Source: CAD feature listing. Evaluate the final solid. Frame: model axes, mm. A direction names the side the tool comes from. Give positions to 0.01 mm unless a question says otherwise; leave off trailing zeros. Write each loop counter-clockwise with the first axis right and the second up, starting at its lowest first coordinate (ties: lowest second). Pieces come first, ordered by that corner, then holes. Notation, with made-up numbers: M 47.25,20 L 69.25,20 A18 cw 69.25,49 Z; hole C 50,7.25 d5. An arc over 180 degrees is marked long. Answer as a JSON object with one key per item and string values. Group by question number.
```python
from build123d import *

# Parameters (mm, degrees)
F0_R          = 5.5
F0_R_2        = 5
F2_DEPTH      = 4
F3_W          = 37.252
F3_H          = 4.7996
F4_DEPTH      = 7.025
F4_DEPTH_BACK = 7.025
F5_T4_DEPTH   = 25.1150634776
F5_T10_DEPTH  = 25.1150634776
F5_T16_DEPTH  = 25.8484060864
F5_T22_DEPTH  = 25.8484060864


# Not quite as in the source:
# - a fillet or chamfer that OpenCascade refuses, or shapes differently, is made with other operations: its cross-section is extruded or revolved along the edge and cut away or added


with BuildPart() as f2:
    # F0 (on Top) → F2 (new body, symmetric)
    with BuildSketch(Plane.XY):
        with BuildLine():
            ThreePointArc((-25.4642125984, 6.5236839855), (-20.8095940807, 4.6358116329), (-18.876, 0))
            ThreePointArc((-18.876, 0), (-20.8095940807, -4.6358116329), (-25.4642125984, -6.5236839855))
            Line((-25.4642125984, -6.5236839855), (25.3308661417, -7.0236597661))
            ThreePointArc((25.3308661417, -7.0236597661), (18.376, 0), (25.3308661417, 7.0236597661))
            Line((25.3308661417, 7.0236597661), (-25.4642125984, 6.5236839855))
        make_face()
        with BuildLine():
            ThreePointArc((32.424, 0), (30.3422150793, 4.9911006913), (25.3308661417, 7.0236597661))
            ThreePointArc((25.3308661417, 7.0236597661), (18.376, 0), (25.3308661417, -7.0236597661))
            ThreePointArc((25.3308661417, -7.0236597661), (30.3422150793, -4.9911006913), (32.424, 0))
        make_face()
        with Locations((25.4, 0)):
            Circle(F0_R, mode=Mode.SUBTRACT)
        with BuildLine():
            ThreePointArc((-25.4642125984, -6.5236839855), (-20.8095940807, -4.6358116329), (-18.876, 0))
            ThreePointArc((-18.876, 0), (-20.8095940807, 4.6358116329), (-25.4642125984, 6.5236839855))
            ThreePointArc((-25.4642125984, 6.5236839855), (-31.924, 0), (-25.4642125984, -6.5236839855))
        make_face()
        with Locations((-25.4, 0)):
            Circle(F0_R_2, mode=Mode.SUBTRACT)
    extrude(amount=F2_DEPTH, both=True)

    # F3 (on Front) → F4 (cut, two sides)
    with BuildSketch(Plane.XZ) as f4_sk:
        with Locations((-0.25, 0)):
            Rectangle(F3_W, F3_H)
    extrude(amount=-F4_DEPTH, mode=Mode.SUBTRACT)
    extrude(f4_sk.sketch, amount=F4_DEPTH_BACK, mode=Mode.SUBTRACT)

    # F5: fillet of radius 2.3876 on 4 edges, made by hand


with BuildPart() as f5_tool2:
    # F5_s3 → F5_t4 (new body)
    with BuildSketch(Plane.XZ.offset(-12.5575317388)):
        with BuildLine():
            ThreePointArc((-18.876, 0.0122), (-18.1766881508, 1.7004881508), (-16.4884, 2.3998))
            Line((-16.4884, 2.3998), (-18.876, 2.3998))
            Line((-18.876, 2.3998), (-18.876, 0.0122))
        make_face()
    extrude(amount=F5_T4_DEPTH)

    split(bisect_by=Plane(origin=(-0.0666732283, 6.7736718758, 0), x_dir=(0, 0, 1), z_dir=(0.0098425197, -0.9999515612, 0)), keep=Keep.TOP)

    split(bisect_by=Plane(origin=(-0.0666732283, -6.7736718758, 0), x_dir=(0, 0, 1), z_dir=(0.0098425197, 0.9999515612, 0)), keep=Keep.TOP)


with BuildPart() as f2_1:
    add(f2.part)

    # F5_t1: union F5_tool2
    add(f5_tool2.part)


with BuildPart() as f5_tool8:
    # F5_s9 → F5_t10 (new body)
    with BuildSketch(Plane.XZ.offset(12.5575317388)):
        with BuildLine():
            ThreePointArc((-16.4884, -2.3998), (-18.1766881508, -1.7004881508), (-18.876, -0.0122))
            Line((-18.876, -0.0122), (-18.876, -2.3998))
            Line((-18.876, -2.3998), (-16.4884, -2.3998))
        make_face()
    extrude(amount=-F5_T10_DEPTH)

    split(bisect_by=Plane(origin=(-0.0666732283, 6.7736718758, 0), x_dir=(0, 0, 1), z_dir=(0.0098425197, -0.9999515612, 0)), keep=Keep.TOP)

    split(bisect_by=Plane(origin=(-0.0666732283, -6.7736718758, 0), x_dir=(0, 0, 1), z_dir=(0.0098425197, 0.9999515612, 0)), keep=Keep.TOP)


with BuildPart() as f2_2:
    add(f2_1.part)

    # F5_t7: union F5_tool8
    add(f5_tool8.part)


with BuildPart() as f5_tool14:
    # F5_s15 → F5_t16 (new body)
    with BuildSketch(Plane.XZ.offset(12.9242030432)):
        with BuildLine():
            ThreePointArc((18.376, -0.0122), (17.6766881508, -1.7004881508), (15.9884, -2.3998))
            Line((15.9884, -2.3998), (18.376, -2.3998))
            Line((18.376, -2.3998), (18.376, -0.0122))
        make_face()
    extrude(amount=-F5_T16_DEPTH)

    split(bisect_by=Plane(origin=(-0.0666732283, 6.7736718758, 0), x_dir=(0, 0, 1), z_dir=(0.0098425197, -0.9999515612, 0)), keep=Keep.TOP)

    split(bisect_by=Plane(origin=(-0.0666732283, -6.7736718758, 0), x_dir=(0, 0, 1), z_dir=(0.0098425197, 0.9999515612, 0)), keep=Keep.TOP)


with BuildPart() as f2_3:
    add(f2_2.part)

    # F5_t13: union F5_tool14
    add(f5_tool14.part)


with BuildPart() as f5_tool20:
    # F5_s21 → F5_t22 (new body)
    with BuildSketch(Plane.XZ.offset(-12.9242030432)):
        with BuildLine():
            ThreePointArc((18.376, 0.0122), (17.6766881508, 1.7004881508), (15.9884, 2.3998))
            Line((15.9884, 2.3998), (18.376, 2.3998))
            Line((18.376, 2.3998), (18.376, 0.0122))
        make_face()
    extrude(amount=F5_T22_DEPTH)

    split(bisect_by=Plane(origin=(-0.0666732283, 6.7736718758, 0), x_dir=(0, 0, 1), z_dir=(0.0098425197, -0.9999515612, 0)), keep=Keep.TOP)

    split(bisect_by=Plane(origin=(-0.0666732283, -6.7736718758, 0), x_dir=(0, 0, 1), z_dir=(0.0098425197, 0.9999515612, 0)), keep=Keep.TOP)


with BuildPart() as f2_4:
    add(f2_3.part)

    # F5_t19: union F5_tool20
    add(f5_tool20.part)


solid = f2_4.part
```
(1) Pull-direction query (X, two-part tool) for faces 3 (the cylindrical face through (-31.922, 0.143, 0.056)), 4 (the flat face through (0, 0, 4)), 5 (the cylindrical face through (-30.395, 0.22, -0.056)); classes: pulls with the +X half, pulls with the -X half, needs draft (parallel to the pull), parting line crosses it, or undercut.
(2) Section C-C, the plane x = 11.5. Return loops of the section in (y, z).
(3) Access query for faces 1 (the cylindrical face through (-18.195, 0.093, 1.682)), 2 (the cylindrical face through (21, -3.3, -0.1)). Directions: +Z, -Z, +X, -X, +Y, -Y. A direction counts if a zero-diameter tool reaches every point of the face in a straight line with its end or side. Return the directions, or none.
(4) Section A-A, the plane y = 0. State how many separate pieces and enclosed holes the cut face has, plus the area to 3 significant figures.
(5) Contact query for flat-ended pins moving along their axis: pin 1 Ø3 at (x, z) = (-11, 1.5) entering from +Y; pin 2 Ø1.5 at (x, z) = (21.5, -2.5) entering from +Y; pin 3 Ø1 at (y, z) = (4.5, 0.5) entering from +X. Output: stop coordinate, or through.
(6) Ray query, L1, parallel to Y at x = -25.4, z = -1.5; L2, parallel to Y at x = 25.4, z = -1.5; L3, parallel to Z at x = 8, y = -2.75. Return the intervals inside material, ascending. Write a range as [from, to].
(7) Section B-B, the plane z = -1. Return loops of the section in (x, y).
Reported:
{
 "1": {"face 3": "pulls with the -X half", "face 4": "needs draft", "face 5": "undercut"},
 "2": {"outline": "M -6.89,-4 L 6.89,-4 L 6.89,-2.4 L -6.89,-2.4 Z; M -6.89,2.4 L 6.89,2.4 L 6.89,4 L -6.89,4 Z"},
 "3": {"face 1": "+Y, -Y", "face 2": "+Z, -Z"},
 "4": {"separate pieces": "3", "enclosed holes": "1", "area": "173 mm2"},
 "5": {"pin 1": "stops at y = 6.68", "pin 2": "stops at y = 6.99", "pin 3": "stops at x = 31.17"},
 "6": {"L1": "y = [-6.52, -5], [5, 6.52]", "L2": "y = [-7.02, -5.5], [5.5, 7.02]", "L3": "z = [-4, -2.4], [2.4, 4]"},
 "7": {"outline": "M -25.46,-6.52 L -18.66,-6.59 L -18.66,6.59 L -25.46,6.52 A6.52 ccw Z; M 18.16,-6.95 L 25.33,-7.02 A7.02 ccw long 25.33,7.02 L 18.16,6.95 Z; hole C -25.4,0 d10; hole C 25.4,0 d11"}
}
